from build123d import *

# Parameters (mm, degrees)
F0_R     = 18.5
F0_R_2   = 0.6
F1_DEPTH = 3
F2_W     = 8.4
F2_H     = 13.5
F3_DEPTH = 4.4
F5_DEPTH = 2.95
F7_DEPTH = 2.95


with BuildPart() as f1:
    # F0 (on Top) → F1 (new body)
    with BuildSketch(Plane.XY):
        Circle(F0_R)
        with Locations((0, -15.5)):
            Circle(F0_R_2, mode=Mode.SUBTRACT)
        with Locations((-15.5, 0)):
            Circle(F0_R_2, mode=Mode.SUBTRACT)
        with Locations((15.5, 0)):
            Circle(F0_R_2, mode=Mode.SUBTRACT)
        with Locations((0, 15.5)):
            Circle(F0_R_2, mode=Mode.SUBTRACT)
    extrude(amount=F1_DEPTH)

    # F2 (on face) → F3 (join)
    with BuildSketch(Plane.XY.offset(3)):
        with Locations((0, 2.25)):
            Rectangle(F2_W, F2_H)
    extrude(amount=F3_DEPTH)

    # F4 (on face) → F5 (cut)
    with BuildSketch(Plane(origin=(-4.2, 0, 0), x_dir=(0, -1, 0), z_dir=(-1, 0, 0))):
        Polygon((-9, 3), (1, 3), (1, 6.1), (-8.229371, 6.1), (-9, 6.503245), align=None)
    extrude(amount=-F5_DEPTH, mode=Mode.SUBTRACT)

    # F6 (on face) → F7 (cut)
    with BuildSketch(Plane.YZ.offset(4.2)):
        Polygon((-0.99, 3), (9, 3), (9, 6.494885), (8.228009, 6.1), (-0.219371, 6.1), (-0.99, 6.1), align=None)
    extrude(amount=-F7_DEPTH, mode=Mode.SUBTRACT)

    # F8 (on face) → F9 (revolve)
    with BuildSketch(Plane.XY.offset(3)):
        with BuildLine():
            Line((2.508028, -8.467954), (-2.508028, -8.467954))
            add(Edge.make_bspline(
                [(-2.508028, -8.467954), (-2.508028, -9.163152), (0, -9.163152), (2.508028, -9.163152), (2.508028, -8.467954)],
                knots=[0, 0, 0, 1.570796, 1.570796, 3.141593, 3.141593, 3.141593], degree=2, weights=[1, 0.707107, 1, 0.707107, 1]))
        make_face()
    revolve(axis=Axis((0, -8.467954, 3), (1, 0, 0)))


solid = f1.part
The listing builds one solid part. Answer for the finished solid, in the listing's coordinates (mm). A direction names the side the tool comes from. Coordinates: 2 decimals unless noted, no trailing zeros. Write each loop counter-clockwise with the first axis right and the second up, starting at its lowest first coordinate (ties: lowest second). Pieces come first, ordered by that corner, then holes. Notation, with made-up numbers: (17, -22.75) - (29, -22.75) arc R17 cw to (29, -14.75) - close; hole circle Ø6 at (49.5, 41.5). An arc over 180 degrees is marked (long way). Return JSON: item names as keys, results as strings.
1. The part is cut by section A-A on y = 0. Determine the outline of the cut face in (x, z).
Final values:
{"outline": "(-18.5, 0) - (-16.1, 0) - (-16.1, 3) - (-18.5, 3) - close; (-14.9, 0) - (14.9, 0) - (14.9, 3) - (1.25, 3) - (1.25, 6.1) - (4.2, 6.1) - (4.2, 7.4) - (-4.2, 7.4) - (-4.2, 6.1) - (-1.25, 6.1) - (-1.25, 3) - (-14.9, 3) - close; (16.1, 0) - (18.5, 0) - (18.5, 3) - (16.1, 3) - close"}
2. For a pull along Y with two mould halves and no side action, classify faces 4 (the face through (-4.01, -18.06, 1.48)), 5 (the face through (16.054, -0.23, 1.479)), 6 (the face through (3, 4, 6.1)), 7 (the face through (-0.078, 16.095, 1.479)) as +Y half, -Y half, draft (parallel to the pull), parting line (faces both ways), or undercut.
Final values:
{"face 4": "parting line", "face 5": "undercut", "face 6": "draft", "face 7": "undercut"}
3. Each of these flat-tipped pins is pushed along its axis until it touches: pin 1 Ø3.5 at (x, z) = (0.5, 5.5) entering from +Y; pin 2 Ø2 at (y, z) = (5, 4.5) entering from +X; pin 3 Ø3 at (x, z) = (9.5, 1.5) entering from -Y. Where does it stop, or does it pass through?
Final values:
{"pin 1": "y = 9", "pin 2": "x = 1.25", "pin 3": "y = -16.68"}
4. Which of the six approach directions +Z, -Z, +X, -X, +Y, -Y give full straight-line access (tool end or side, diameter ignored) to faces 1 (the face through (0, 9, 6)), 2 (the face through (-3, -1, 5)), 3 (the face through (4.2, 1, 7))?
Final values:
{"face 1": "+Z, +X, -X, +Y", "face 2": "-X, +Y", "face 3": "+Z, +X, +Y, -Y"}
5. Consider line 1 along Y through (x, z) = (0, 2.05); line 2 along Z through (x, y) = (-4, 2); line 3 along Z through (x, y) = (6.5, -12.5). Determine where each line is inside the solid, lowest interval first.
Final values:
{"line 1": "-18.5 to -16.1, -14.9 to 14.9, 16.1 to 18.5", "line 2": "0 to 3, 6.1 to 7.4", "line 3": "0 to 3"}
6. The part is cut by section B-B on x = 15.5. Determine the outline of the cut face in (y, z).
Final values:
{"outline": "(-10.1, 0) - (-0.6, 0) - (-0.6, 3) - (-10.1, 3) - close; (0.6, 0) - (10.1, 0) - (10.1, 3) - (0.6, 3) - close"}
7. The part is cut by section C-C on z = 1.5. Determine the outline of the cut face in (x, y), then the cut area to 3 significant figures.
Final values:
{"outline": "circle Ø37 at (0, 0); hole circle Ø1.2 at (-15.5, 0); hole circle Ø1.2 at (0, -15.5); hole circle Ø1.2 at (0, 15.5); hole circle Ø1.2 at (15.5, 0)", "area": "1,070 mm^2"}
8. The part is cut by section D-D on x = 0. Count the separate pieces of the cut face and the enclosed holes in it, then the cut area to 3 significant figures.
Final values:
{"separate pieces": "3", "enclosed holes": "0", "area": "164 mm^2"}
